Verification items for the finished model (mm, model axes). A direction names the side the tool comes from. Round coordinates to 2 decimals unless told otherwise and drop trailing zeros. Order: outer loops, then holes, each group sorted by start corner. A loop starts at its lowest first (then second) coordinate and runs counter-clockwise, first axis right, second up. Notation, with made-up numbers: M -22.75,52 L -1.75,52 A17 ccw -1.75,71 Z; hole C 21,-20.5 d11. An arc over 180 degrees is marked long. Write item = value, one per line. Start each with the question number.
from build123d import *

# Parameters (mm, degrees)
F1_DEPTH = 25.4
F3_DEPTH = 25.4


with BuildPart() as f1:
    # F0 (on Top) → F1 (new body)
    with BuildSketch(Plane.XY):
        Polygon((-170.958579, 12.585102), (-98.389238, 25.517641), (-149.032265, -57.078436), (-108.417206, -112.903006), (-77.047296, -4.846431), (-74.092499, 5.331642), (-51.749377, 5.331642), (-51.749377, 12.585102), (106.318571, 5.331642), (96.669301, 57.336546), (36.629643, 62.309485), (-59.037734, 69.580153), (-113.755345, 75.21973), (-182.120658, 75.21973), align=None)
        Polygon((-74.092499, 5.331642), (-77.047296, -4.846431), (-63.583464, -8.755117), (-54.704174, -4.846431), (-51.749377, 5.331642), align=None)
    extrude(amount=F1_DEPTH)

    # F2 (on face) → F3 (join)
    with BuildSketch(Plane.XY.offset(25.4)):
        Polygon((-54.704174, 12.585102), (-72.897859, 11.73104), (-77.047296, 0), (-63.345755, -4.846431), (-59.143819, 0), align=None)
    extrude(amount=F3_DEPTH)


solid = f1.part
1) Gauge pin test, flat ends, axial feed: P1, Ø3.5, axis at y = 10.5, z = 10.5, coming from the +X side; P2, Ø1.5, axis at x = -114.5, y = 0, coming from the +Z side; P3, Ø8, axis at y = 10, z = 7.5, coming from the -X side. Record the tip position at first contact, or that the pin passes through.
2) Cross-section at B-B, the plane y = 16. Enter the section's corners in (x, z).
3) Cross-section at A-A, the plane x = -137.5. Enter the section's corners in (y, z), then the cut area to 3 significant figures.
4) Cross-section at D-D, the plane z = 21.5. Enter the section's corners in (x, y).
5) Cross-section at C-C, the plane z = 40.5. Enter the section's corners in (x, y), then the cut area to 3 significant figures.
6) Scan lines: probe 1 along Z at (x, y) = (-56, -2); probe 2 along Y at (x, z) = (-127.5, 2); probe 3 along Y at (x, z) = (-75, 25). Record each from-to range of solid material in increasing order.
7) Release check for a two-part mould opening along X. For faces 6 (the flat face through (-70.41, -6.773, 12.522)), 7 (the flat face through (-74.944, 5.948, 37.922)), 8 (the flat face through (-59.21, -6.83, 12.52)) record: pulls with the +X half, pulls with the -X half, needs draft (parallel to the pull), parting line crosses it, or undercut.
8) Access from +Z, -Z, +X, -X, +Y, -Y to the whole of each face (thin tool, end or side, straight path). Record for faces 1 (the flat face through (26.18, 9.01, 12.52)), 2 (the flat face through (-135.18, 18.96, 12.52)), 3 (the flat face through (-176.618, 44.341, 12.522)), 4 (the flat face through (-70.29, -2.39, 37.92)), 5 (the flat face through (-63.674, 12.164, 37.922)).
Geometry results:
q1.P1 = 105.68
q1.P2 = 25.4
q1.P3 = -171.21
q2.outline = M -171.57,0 L -151.8,0 L -151.8,25.4 L -171.57,25.4 Z; M -104.22,0 L 104.34,0 L 104.34,25.4 L -104.22,25.4 Z
q3.outline = M -72.93,0 L -38.27,0 L -38.27,25.4 L -72.93,25.4 Z; M 18.55,0 L 75.22,0 L 75.22,25.4 L 18.55,25.4 Z
q3.area = 2,320 mm^2
q4.outline = M -182.12,75.22 L -170.96,12.59 L -98.39,25.52 L -149.03,-57.08 L -108.42,-112.9 L -77.05,-4.85 L -63.58,-8.76 L -54.7,-4.85 L -51.75,5.33 L -51.75,12.59 L 106.32,5.33 L 96.67,57.34 L 36.63,62.31 L -59.04,69.58 L -113.76,75.22 Z
q5.outline = M -77.05,0 L -63.35,-4.85 L -59.14,0 L -54.7,12.59 L -72.9,11.73 Z
q5.area = 261 mm^2
q6.probe_1 = 0 to 25.4
q6.probe_2 = -86.67 to -21.96, 20.33 to 75.22
q6.probe_3 = -5.44 to 71.23
q7.face_6 = undercut
q7.face_7 = pulls with the -X half
q7.face_8 = pulls with the +X half
q8.face_1 = +Z, -Z, -Y
q8.face_2 = +Z, -Z
q8.face_3 = +Z, -Z, -X, -Y
q8.face_4 = +Z, -X, -Y
q8.face_5 = +Z, -X, +Y
